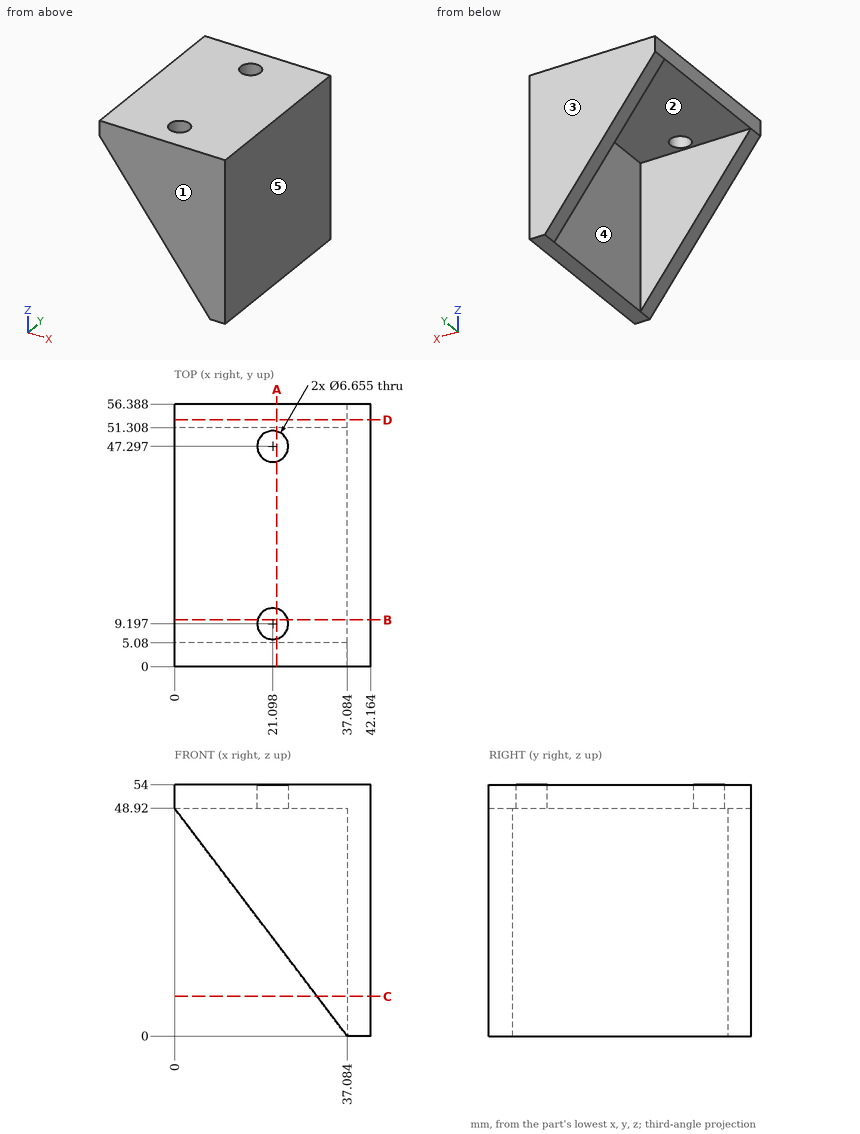
The figure shows three views and two pictorial views of one solid part (mm, origin at its lowest corner). Answer the questions. A direction names the side the tool comes from. Give positions to 0.01 mm unless a question says otherwise; leave off trailing zeros. Write each loop counter-clockwise with the first axis right and the second up, starting at its lowest first coordinate (ties: lowest second). Pieces come first, ordered by that corner, then holes. Notation, with made-up numbers: (-27.5, 63) -> (-9.5, 63) arc R30 cw to (-9.5, 90) -> close; hole circle Ø11 at (75.25, 55). An arc over 180 degrees is marked (long way). Use one line per item in the form item = value.
1) Section C-C on z = 8.5 is taken. Write down the section's boundary in (x, y).
Result:
outline = (30.64, 0) -> (42.16, 0) -> (42.16, 56.39) -> (30.64, 56.39) -> (30.64, 51.31) -> (37.08, 51.31) -> (37.08, 5.08) -> (30.64, 5.08) -> close
2) Section D-D on y = 53 is taken. Write down the section's boundary in (x, z).
Result:
outline = (0, 48.92) -> (37.08, 0) -> (42.16, 0) -> (42.16, 54) -> (0, 54) -> close
3) A tool of negligible diameter and unlimited length cuts with its end or side. For the marked faces 4 and 5, from which of +Z, -Z, +X, -X, +Y, -Y can it reach the whole face along a straight path? Write none if from no direction.
Result:
face_4 = -Z, -X
face_5 = +Z, -Z, +X, +Y, -Y
4) Section B-B on y = 10 is taken. Write down the section's boundary in (x, z).
Result:
outline = (0, 48.92) -> (17.87, 48.92) -> (17.87, 54) -> (0, 54) -> close; (24.33, 48.92) -> (37.08, 48.92) -> (37.08, 0) -> (42.16, 0) -> (42.16, 54) -> (24.33, 54) -> close
5) Section A-A on x = 22 is taken. Write down the section's boundary in (y, z), plus the area to 3 significant figures.
Result:
outline = (0, 19.9) -> (5.08, 19.9) -> (5.08, 48.92) -> (5.99, 48.92) -> (5.99, 54) -> (0, 54) -> close; (12.4, 48.92) -> (44.09, 48.92) -> (44.09, 54) -> (12.4, 54) -> close; (50.5, 48.92) -> (51.31, 48.92) -> (51.31, 19.9) -> (56.39, 19.9) -> (56.39, 54) -> (50.5, 54) -> close
area = 516 mm²
6) Each of these flat-tipped pins is pushed along its axis until it touches: P1, Ø8, axis at y = 12.5, z = 28.5, coming from the -X side; P2, Ø5.5, axis at x = 21.1, y = 47.3, coming from the -Z side; P3, Ø7.5, axis at x = 21.1, y = 9.2, coming from the -Z side. Where does it stop, or does it pass through?
Result:
P1 = 37.08
P2 = through
P3 = 48.92
7) For a pull along Y with two mould halves and no side action, classify the marked faces 1, 2 and 3 as +Y half, -Y half, draft (parallel to the pull), parting line (faces both ways), or undercut.
Result:
face_1 = -Y half
face_2 = undercut
face_3 = +Y half
8) Straight lines are drawn through the part: probe 1 along Z at (x, y) = (28.5, 34.5); probe 2 along X at (y, z) = (35, 48); probe 3 along X at (y, z) = (52, 6) (1 decimal). For each, find the intervals that lie inside material, in ascending order.
Result:
probe_1 = 48.92 to 54
probe_2 = 37.08 to 42.16
probe_3 = 32.5 to 42.2
